Work out the finished part from the listing and answer in its coordinate system (mm). Face numbers are marked on the shaded views. A direction names the side the tool comes from. Coordinates: 2 decimals unless noted, no trailing zeros. Use CSV: the item, a comma, the result in double quotes.
from build123d import *

# Parameters (mm, degrees)
F0_W      = 15
F0_H      = 3
F0_W_2    = 1.5
F0_H_2    = 26
F0_W_3    = 2.5
F1_DEPTH  = 3.5
F2_R      = 3.5
F3_DEPTH  = 9
F4_R      = 1
F5_R      = 3
F6_R      = 2
F7_R      = 1
F8_SIZE2  = 1.99999
F8_SIZE   = 6.99999
F9_W      = 4
F9_H      = 26
F10_DEPTH = 4


# Not quite as in the source:
# - a fillet or chamfer is up to 0.001 mm smaller than in the source, because OpenCascade refuses the exact size


with BuildPart() as f1:
    # F0 (on Right) → F1 (new body, symmetric)
    with BuildSketch(Plane.YZ):
        with Locations((-4.5, 6)):
            Rectangle(F0_W, F0_H)
        Polygon((-12, -4.5), (-12, 4.5), (-12, 7.5), (-12, 16), (-27, 16), (-27, -16), (-12, -16), (-12, -7.5), align=None)
        with Locations((-22.25, 0)):
            Rectangle(F0_W_2, F0_H_2, mode=Mode.SUBTRACT)
        with Locations((-16.25, 0)):
            Rectangle(F0_W_3, F0_H_2, mode=Mode.SUBTRACT)
        with Locations((-4.5, -6)):
            Rectangle(F0_W, F0_H)
    extrude(amount=F1_DEPTH, both=True)

    # F2 (on face) → F3 (join, through all)
    with BuildSketch(Plane.XY.offset(-4.5)):
        Circle(F2_R)
    extrude(amount=F3_DEPTH)

    # F4
    f4_edges = [f1.edges().sort_by_distance(p)[0] for p in [
        (0, -27, 16),
        (0, -12, 16),
        (0, -27, -16),
        (0, -12, -16),
    ]]
    fillet(f4_edges, radius=F4_R)

    # F5
    f5_edges = [f1.edges().sort_by_distance(p)[0] for p in [
        (0, -12, 7.5),
        (0, -12, -7.5),
    ]]
    fillet(f5_edges, radius=F5_R)

    # F6
    f6_edges = [f1.edges().sort_by_distance(p)[0] for p in [
        (0, 3, 7.5),
        (0, 3, -7.5),
        (0, -12, -4.5),
        (0, -12, 4.5),
    ]]
    fillet(f6_edges, radius=F6_R)

    # F7
    f7_edges = [f1.edges().sort_by_distance(p)[0] for p in [
        (-3.5, -4, -7.5),
        (-3.5, -4, 7.5),
        (3.5, 2.414214, 6.914214),
        (3.5, 2.414214, -6.914214),
    ]]
    fillet(f7_edges, radius=F7_R)

    # F8 (size 7 and 2 in the source; OpenCascade refuses exactly that, so slightly less here)
    f8_edges = [f1.edges().sort_by_distance(p)[0] for p in [
        (3.5, -23, 0),
    ]]
    f8_side = f1.faces().sort_by_distance((0, -23, 0))[0]
    chamfer(f8_edges, length=F8_SIZE, length2=F8_SIZE2, reference=f8_side)

    # F9 (on face) → F10 (cut)
    with BuildSketch(Plane(origin=(-3.5, 0, 0), x_dir=(0, -1, 0), z_dir=(-1, 0, 0))):
        with Locations((19.5, 0)):
            Rectangle(F9_W, F9_H)
    extrude(amount=-F10_DEPTH, mode=Mode.SUBTRACT)


solid = f1.part
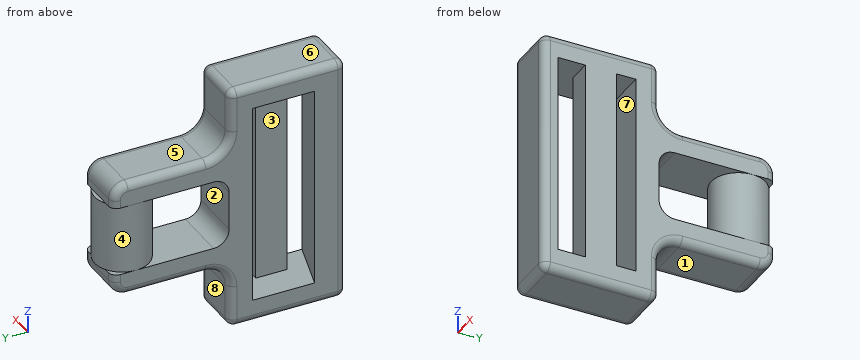
Item 1: Given pin 1 (0.8 mm diameter, centred on x = 2.5, y = 1, fed in from +Z); pin 2 (0.5 mm diameter, centred on x = -2.5, y = 1.5, fed in from -Z); pin 3 (0.6 mm diameter, centred on x = 0.5, y = 3.5, fed in from -Z), each flat-ended and moving along its own axis, determine where each tip first touches the part or whether it passes through.
Answer:
pin 1,"stops at z = 7.5"
pin 2,"stops at z = -7.48"
pin 3,"stops at z = -4.5"
Item 2: The part is cut by section A-A (z = 12). Count the separate pieces of the cut face and the enclosed holes in it, then the cut area to 3 significant figures.
Answer:
separate pieces,"3"
enclosed holes,"0"
area,"53.1 mm2"
Item 3: Consider probe 1 along Y at (x, z) = (1.5, 12); probe 2 along Y at (x, z) = (3, 11.5); probe 3 along Y at (x, z) = (1.5, 2). Determine where each line is inside the solid, lowest interval first.
Answer:
probe 1,"y = -27 to -24.43, -21.5 to -17.5, -15 to -12"
probe 2,"y = -26.87 to -24.86, -21.5 to -17.5, -15 to -12.13"
probe 3,"y = -27 to -24.43, -21.5 to -17.5, -15 to -12, -3.16 to 3.16"
Item 4: A tool of negligible diameter and unlimited length cuts with its end or side. For the marked faces 1, 2, 3, 4 and 5, from which of +Z, -Z, +X, -X, +Y, -Y can it reach the whole face along a straight path? Write none if from no direction.
Answer:
face 1,"-Z, +X, -X, +Y"
face 2,"+X, -X"
face 3,"-X"
face 4,"none"
face 5,"+Z, +X, -X, +Y"
Item 5: For a pull along Z with two mould halves and no side action, classify the marked faces 6, 7 and 8 as released by +Z, released by -Z, zero draft, split by the parting line, or undercut.
Answer:
face 6,"released by +Z"
face 7,"undercut"
face 8,"zero draft"
